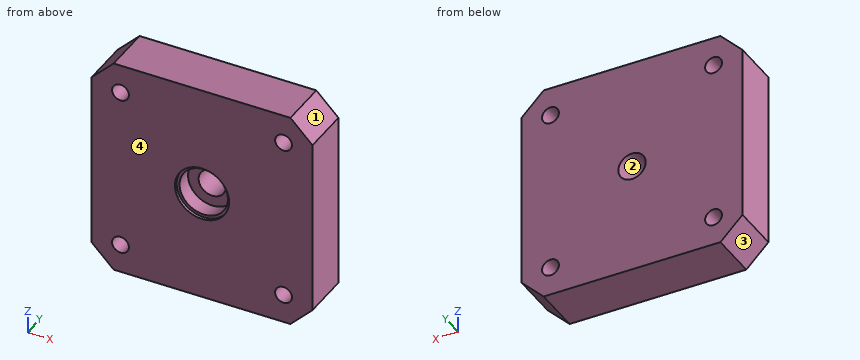
```python
from build123d import *

# Parameters (mm, degrees)
SKETCH_1_W          = 42
SKETCH_1_H          = 42
SKETCH_1_R          = 1.6
SKETCH_1_R_2        = 2.6
EXTRUDE_1_DEPTH     = 9.15
SKETCH_2_R          = 5.15
CUT_EXTRUDE_1_DEPTH = 0.6
CHAMFER_1_SIZE      = 4.2
SKETCH_3_R          = 4.6
CUT_EXTRUDE_2_DEPTH = 3


with BuildPart() as part:
    # 草图1 → 凸台-拉伸1 (new body)
    with BuildSketch(Plane(origin=(0, 0, 0), x_dir=(1, 0, 0), z_dir=(0, 1, 0))):
        Rectangle(SKETCH_1_W, SKETCH_1_H)
        with Locations((-15.5, 15.5)):
            Circle(SKETCH_1_R, mode=Mode.SUBTRACT)
        with Locations((15.5, 15.5)):
            Circle(SKETCH_1_R, mode=Mode.SUBTRACT)
        with Locations((15.5, -15.5)):
            Circle(SKETCH_1_R, mode=Mode.SUBTRACT)
        with Locations((-15.5, -15.5)):
            Circle(SKETCH_1_R, mode=Mode.SUBTRACT)
        Circle(SKETCH_1_R_2, mode=Mode.SUBTRACT)
    extrude(amount=EXTRUDE_1_DEPTH)

    # 草图2 → 切除-拉伸1 (cut)
    with BuildSketch(Plane.XZ):
        Circle(SKETCH_2_R)
    extrude(amount=-CUT_EXTRUDE_1_DEPTH, mode=Mode.SUBTRACT)

    # 倒角1
    chamfer_1_edges = [part.edges().sort_by_distance(p)[0] for p in [
        (21, 4.575, 21),
        (-21, 4.575, 21),
        (-21, 4.575, -21),
        (21, 4.575, -21),
    ]]
    chamfer(chamfer_1_edges, length=CHAMFER_1_SIZE)

    # 草图3 → 切除-拉伸2 (cut)
    with BuildSketch(Plane.XZ.offset(-0.6)):
        Circle(SKETCH_3_R)
    extrude(amount=-CUT_EXTRUDE_2_DEPTH, mode=Mode.SUBTRACT)


solid = part.part
```
Here's how the part is built. I have some questions about the finished solid (model axes, mm). Face numbers are marked on the shaded views. Coordinates: 2 decimals unless noted, no trailing zeros. Order: outer loops, then holes, each group sorted by start corner. A loop starts at its lowest first (then second) coordinate and runs counter-clockwise, first axis right, second up. Notation, with made-up numbers: (-40, 65) - (14, 65) arc R29 ccw to (14, 99) - close; hole circle Ø2 at (-30.75, 87.25). An arc over 180 degrees is marked (long way). One line per question, with ' | ' between items.
(1) Will these pins go through, and if not, where does the flat tip stop? pin 1 (5 mm diameter, centred on x = 2.5, z = 0.5, fed in from -Y); pin 2 (4.5 mm diameter, centred on x = -1, z = 1, fed in from -Y).
Report:
pin 1: stops at y = 0.6 | pin 2: stops at y = 3.6
(2) If we mould it in two halves opening along X, with no side actions, what happens to the marked faces 1, 2, 3 and 4? For each: pulls with the +X half, pulls with the -X half, needs draft (parallel to the pull), parting line crosses it, or undercut.
Report:
face 1: pulls with the +X half | face 2: undercut | face 3: pulls with the -X half | face 4: needs draft
(3) Suppose I cut it at D-D on x = -15.5. List the corners of the cut face in (y, z) for me, and give its area (3 significant figures).
Report:
outline: (0, -21) - (9.15, -21) - (9.15, -17.1) - (0, -17.1) - close; (0, -13.9) - (9.15, -13.9) - (9.15, 13.9) - (0, 13.9) - close; (0, 17.1) - (9.15, 17.1) - (9.15, 21) - (0, 21) - close | area: 326 mm2
(4) If I drill on L1, parallel to X at y = 4.75, z = -15.5; L2, parallel to X at y = 6.2, z = 0, over which ranges is the centre line in solid material (lowest first)?
Report:
L1: x = -21 to -17.1, -13.9 to 13.9, 17.1 to 21 | L2: x = -21 to -2.6, 2.6 to 21
(5) Suppose I cut it at A-A on z = 15.5. List the corners of the cut face in (x, y) for me.
Report:
outline: (-21, 0) - (-17.1, 0) - (-17.1, 9.15) - (-21, 9.15) - close; (-13.9, 0) - (13.9, 0) - (13.9, 9.15) - (-13.9, 9.15) - close; (17.1, 0) - (21, 0) - (21, 9.15) - (17.1, 9.15) - close
(6) Suppose I cut it at C-C on z = 0. List the corners of the cut face in (x, y) for me.
Report:
outline: (-21, 0) - (-5.15, 0) - (-5.15, 0.6) - (-4.6, 0.6) - (-4.6, 3.6) - (-2.6, 3.6) - (-2.6, 9.15) - (-21, 9.15) - close; (2.6, 3.6) - (4.6, 3.6) - (4.6, 0.6) - (5.15, 0.6) - (5.15, 0) - (21, 0) - (21, 9.15) - (2.6, 9.15) - close
(7) Suppose I cut it at B-B on x = 0. List the corners of the cut face in (y, z) for me.
Report:
outline: (0, -21) - (9.15, -21) - (9.15, -2.6) - (3.6, -2.6) - (3.6, -4.6) - (0.6, -4.6) - (0.6, -5.15) - (0, -5.15) - close; (0, 5.15) - (0.6, 5.15) - (0.6, 4.6) - (3.6, 4.6) - (3.6, 2.6) - (9.15, 2.6) - (9.15, 21) - (0, 21) - close
